For this review, take the finished solid that the model builds, in its own axes (mm). A direction names the side the tool comes from. Round coordinates to 2 decimals unless told otherwise and drop trailing zeros. Write each loop counter-clockwise with the first axis right and the second up, starting at its lowest first coordinate (ties: lowest second). Pieces come first, ordered by that corner, then holes. Notation, with made-up numbers: M -24.5,-30.5 L 31.5,-30.5 A11 ccw 31.5,-15.5 Z; hole C -34.75,71.5 d1. An arc over 180 degrees is marked long. Write each question's results on one line, items separated by ' | '. Start each with the question number.
```python
from build123d import *

# Parameters (mm, degrees)
SKETCH1_R           = 1.5
SKETCH1_W           = 42
SKETCH1_H           = 20
BOSS_EXTRUDE1_DEPTH = 3
FILLET1_R           = 5


with BuildPart() as part:
    # Sketch1 → Boss-Extrude1 (new body)
    with BuildSketch(Plane(origin=(0, 0, 0), x_dir=(0, 0, -1), z_dir=(1, 0, 0))):
        Polygon((-33, 0), (-32, 48), (25, 48), (26, 0), (26, -3), (19, -3), (19, 0), (13, 0), (13, -3), (6, -3), (6, 0), (0, 0), (0, -3), (-7, -3), (-7, 0), (-13, 0), (-13, -3), (-20, -3), (-20, 0), (-26, 0), (-26, -3), (-33, -3), align=None)
        with Locations((21.65, 34.9)):
            Circle(SKETCH1_R, mode=Mode.SUBTRACT)
        with Locations(Location((21.65, 25.1, 0), (0, 0, 180))):
            Circle(SKETCH1_R, mode=Mode.SUBTRACT)
        with Locations(Location((-28.65, 34.9, 0), (0, 0, 180))):
            Circle(SKETCH1_R, mode=Mode.SUBTRACT)
        with Locations((-28.65, 25.1)):
            Circle(SKETCH1_R, mode=Mode.SUBTRACT)
        with Locations((-3.5, 30)):
            Rectangle(SKETCH1_W, SKETCH1_H, mode=Mode.SUBTRACT)
    extrude(amount=BOSS_EXTRUDE1_DEPTH)

    # Fillet1
    fillet1_edges = [part.edges().sort_by_distance(p)[0] for p in [
        (1.5, 48, 32),
        (1.5, 48, -25),
    ]]
    fillet(fillet1_edges, radius=FILLET1_R)


solid = part.part
```
Item 1: For faces 4 (the flat face through (1, -1, 26)), 5 (the flat face through (1, 40, 4)), 6 (the flat face through (0, 17, 3)), list the 3-axis set-ups (+Z, -Z, +X, -X, +Y, -Y) from which the entire face can be reached by the end or side of a thin tool; tool diameter is ignored.
Item 2: We need section C-C on x = 1.6. State how many separate pieces and enclosed holes the cut face has, then the cut area to 3 significant figures.
Item 3: We need section B-B on y = 38.5. State the section outline as (x, z) points, then the cut area to 3 significant figures.
Item 4: We need section D-D on y = 25.1. State the section outline as (x, z) points, then the cut area to 3 significant figures.
Item 5: Insertion check: P1, Ø1.5, axis at x = 0.5, y = 3.5, coming from the +Z side; P2, Ø1.5, axis at x = 1, z = -1.5, coming from the -Y side. Each pin has a flat end and moves straight along its axis. Give the tip position at first contact, or say it passes through.
Item 6: Mouldability with a two-part tool opening along Z and no side actions: class faces 1 (the flat face through (1, -3, -23)), 2 (the flat face through (1, -2, 7)), 3 (the cylindrical face through (1.521, 46.534, 30.64)) as pulls with the +Z half, pulls with the -Z half, needs draft (parallel to the pull), parting line crosses it, or undercut.
Item 7: For probe 1 along Y at (x, z) = (2, -11); probe 2 along Y at (x, z) = (1.4, -3.5); probe 3 along Y at (x, z) = (2.6, -22), list the stretches that pass through material, from the lowest coordinate up.
Item 8: We need section A-A on z = -16. State the section outline as (x, y) points, then the cut area to 3 significant figures.
Numbers:
1) face 4: +X, -X, -Y | face 5: +X, -X | face 6: +Z, -Z, -X, +Y, -Y
2) separate pieces: 1 | enclosed holes: 5 | area: 2,010 mm^2
3) outline: M 0,-25.2 L 3,-25.2 L 3,-17.5 L 0,-17.5 Z; M 0,24.5 L 3,24.5 L 3,32.2 L 0,32.2 Z | area: 46.2 mm^2
4) outline: M 0,-25.48 L 3,-25.48 L 3,-23.15 L 0,-23.15 Z; M 0,-20.15 L 3,-20.15 L 3,-17.5 L 0,-17.5 Z; M 0,24.5 L 3,24.5 L 3,27.15 L 0,27.15 Z; M 0,30.15 L 3,30.15 L 3,32.48 L 0,32.48 Z | area: 29.9 mm^2
5) P1: stops at z = 32.94 | P2: stops at y = 0
6) face 1: needs draft | face 2: undercut | face 3: pulls with the +Z half
7) probe 1: y = -3 to 20, 40 to 48 | probe 2: y = 0 to 20, 40 to 48 | probe 3: y = -3 to 23.64, 26.56 to 33.44, 36.36 to 47.63
8) outline: M 0,0 L 3,0 L 3,20 L 0,20 Z; M 0,40 L 3,40 L 3,48 L 0,48 Z | area: 84.0 mm^2
